```python
from build123d import *

# Parameters (mm, degrees)
SKETCH2_R           = 2.1
BOSS_EXTRUDE1_DEPTH = 4
BOSS_EXTRUDE2_DEPTH = 2
CHAMFER1_SIZE       = 30
CHAMFER1_SIZE2      = 3.683536827087146
FILLET2_R           = 1.5
FILLET4_R           = 1.5


with BuildPart() as part:
    # Sketch2 → Boss-Extrude1 (new body)
    with BuildSketch(Plane(origin=(0, 0, 0), x_dir=(1, 0, 0), z_dir=(0, 1, 0))):
        with BuildLine():
            Line((-4.4, -1.507e-14), (-4.4, 12))
            ThreePointArc((-4.4, 12), (2.7e-16, 16.4), (4.4, 12))
            Line((4.4, 12), (4.4, 1.507e-14))
            Line((4.4, 1.507e-14), (4.4, -38.000000000000014))
            Line((4.4, -38.000000000000014), (-4.399999999999994, -38.000000000000014))
            Line((-4.399999999999994, -38.000000000000014), (-4.4, -1.507e-14))
        make_face()
        with Locations(Location((0, 5, 0), (0, 0, 270))):
            Circle(SKETCH2_R, mode=Mode.SUBTRACT)
    extrude(amount=BOSS_EXTRUDE1_DEPTH)

    # Sketch3 → Boss-Extrude2 (add)
    with BuildSketch(Plane(origin=(0, 4, 0), x_dir=(1, 0, 0), z_dir=(0, 1, 0))):
        Polygon((-12, 0), (12, 0), (12.000000000000002, -38), (-11.999999999999995, -38), align=None)
    extrude(amount=BOSS_EXTRUDE2_DEPTH)

    # Chamfer1
    chamfer1_edges = [part.edges().sort_by_distance(p)[0] for p in [
        (3.55e-15, 0, 38.000000000000014),
    ]]
    chamfer1_side = [part.faces().sort_by_distance(p)[0] for p in [
        (1.53e-15, 0, 11.756614981879217),
    ]]
    chamfer(chamfer1_edges, length=CHAMFER1_SIZE, length2=CHAMFER1_SIZE2, reference=chamfer1_side[0])

    # Fillet2
    # the kernel refuses this fillet: 1.5 mm, written as the material it adds along each edge
    with BuildSketch(Plane(origin=(-4.399999999999994, 4, 38.000000000000014), x_dir=(-4.14e-15, -1, 0), z_dir=(-1.2e-16, 0, -1))) as fillet2_piece_1_section:
        with BuildLine():
            CenterArc((FILLET2_R, FILLET2_R), FILLET2_R, 180, 89.99999999999977)
            Line((6.22e-15, FILLET2_R), (0, 0))
            Line((0, 0), (FILLET2_R, 0))
        make_face()
    fillet2_piece_1 = extrude(amount=38.000000000000014, mode=Mode.PRIVATE)
    fillet2_piece_1 = split(fillet2_piece_1, bisect_by=Plane(origin=(-4.741166225178414, 1.3298279167086908, 18.830579243267316), z_dir=(0, 0.992546151641322, -0.12186934340514775)), keep=Keep.TOP, mode=Mode.PRIVATE)
    add(fillet2_piece_1)
    with BuildSketch(Plane(origin=(4.4, 4, 0), x_dir=(0, -1, 0), z_dir=(0, 0, 1))) as fillet2_piece_2_section:
        with BuildLine():
            CenterArc((FILLET2_R, FILLET2_R), FILLET2_R, 180, 90)
            Line((0, FILLET2_R), (0, 0))
            Line((0, 0), (FILLET2_R, 0))
        make_face()
    fillet2_piece_2 = extrude(amount=38.000000000000014, mode=Mode.PRIVATE)
    fillet2_piece_2 = split(fillet2_piece_2, bisect_by=Plane(origin=(4.741166225178429, 1.3298279167086202, 18.830579243266737), z_dir=(0, 0.992546151641322, -0.12186934340514775)), keep=Keep.TOP, mode=Mode.PRIVATE)
    add(fillet2_piece_2)
    # the kernel refuses this fillet: 1.5 mm, written as the material it takes off along each edge
    with BuildSketch(Plane(origin=(-11.999999999999995, 4, 41.75), x_dir=(0, 1, 0), z_dir=(-1.4e-16, 0, -1))) as fillet2_2_piece_1:
        with BuildLine():
            CenterArc((FILLET2_R, FILLET2_R), FILLET2_R, 180, 90)
            Line((0, FILLET2_R), (0, 0))
            Line((0, 0), (FILLET2_R, 0))
        make_face()
    extrude(amount=45.5, mode=Mode.SUBTRACT)
    with BuildSketch(Plane(origin=(12, 4, -3.75), x_dir=(-1, 0, 5e-17), z_dir=(5e-17, 0, 1))) as fillet2_2_piece_2:
        with BuildLine():
            CenterArc((FILLET2_R, -FILLET2_R), FILLET2_R, 90, 90)
            Line((0, -FILLET2_R), (0, 0))
            Line((0, 0), (FILLET2_R, 0))
        make_face()
    extrude(amount=45.5, mode=Mode.SUBTRACT)

    # Fillet4
    fillet4_edges = [part.edges().sort_by_distance(p)[0] for p in [
        (5.41281689306181, 3.918679886483928, 38),
        (8.2, 4, 38),
        (11.560660171779821, 4.439339828220179, 38),
        (-5.41281689306181, 3.918679886483928, 38),
        (-8.200000000000001, 4, 38),
        (-11.560660171779821, 4.439339828220179, 38),
        (12.000000000000002, 5.75, 38),
        (-11.999999999999995, 5.75, 38),
    ]]
    fillet(fillet4_edges, radius=FILLET4_R)


solid = part.part
```
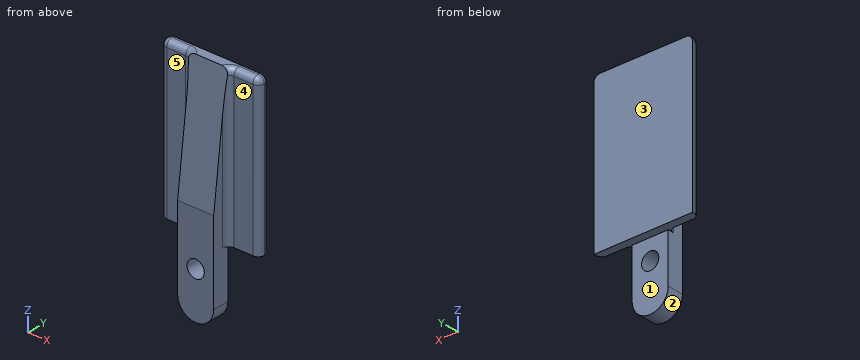
Work out the finished part from the listing and answer in its coordinate system (mm). Face numbers are marked on the shaded views. A direction names the side the tool comes from. Round coordinates to 2 decimals unless told otherwise and drop trailing zeros. Loops run counter-clockwise (first coordinate to the right, second up) from the corner with the lowest first, then second, coordinate; pieces in that order, holes last. Notation, with made-up numbers: (55, -9) -> (76, -9) arc R14 ccw to (76, 11) -> close; hole circle Ø6 at (4, 75). An arc over 180 degrees is marked (long way). Write each question's results on one line, items separated by ' | '. Start each with the question number.
1. Section A-A (x = 0) is taken. Determine the outline of the cut face in (y, z), plus the area to 3 significant figures.
2. A tool of negligible diameter and unlimited length cuts with its end or side. For the marked faces 1, 2, 3, 4 and 5, from which of +Z, -Z, +X, -X, +Y, -Y can it reach the whole face along a straight path? Write none if from no direction.
3. Find the intervals of material crossed by probe 1 along X at (y, z) = (2.35, -5); probe 2 along Y at (x, z) = (-7.5, 18.5); probe 3 along X at (y, z) = (3.5, 2), in increasing order. Write a range as from..to.
4. Section D-D (y = 0.5) is taken. Determine the outline of the cut face in (x, z).
5. Section B-B (z = -5) is taken. Determine the outline of the cut face in (x, y).
6. Section C-C (z = 10) is taken. Determine the outline of the cut face in (x, y).
7. Given pin 1 Ø2.5 at (x, z) = (8.5, 14.5) entering from -Y; pin 2 Ø3 at (x, y) = (6, 1) entering from -Z; pin 3 Ø1 at (x, y) = (-6, 4.5) entering from -Z; pin 4 Ø10 at (x, z) = (6.5, 16) entering from -Y, each flat-ended and moving along its own axis, determine where each tip first touches the part or whether it passes through.
Evaluation:
1) outline: (0, -16.4) -> (4, -16.4) -> (4, -7.1) -> (0, -7.1) -> close; (0, -2.9) -> (4, -2.9) -> (4, 0) -> (6, 0) -> (6, 38) -> (3.68, 38) -> (0, 8) -> close | area: 222 mm2
2) face 1: -Z, +X, -X, +Y | face 2: -Z, +Y, -Y | face 3: +Z, -Z, +X, -X, +Y | face 4: +Z, -Z, +X, -Y | face 5: +Z, -Z, -X, -Y
3) probe 1: x = -4.4..-2.1, 2.1..4.4 | probe 2: y = 4..6 | probe 3: x = -4.78..4.78
4) outline: (-4.4, -12) arc R4.4 ccw to (4.4, -12) -> (4.4, 12.07) -> (-4.4, 12.07) -> close; hole circle Ø4.2 at (0, -5)
5) outline: (-4.4, 0) -> (-2.1, 0) -> (-2.1, 4) -> (-4.4, 4) -> close; (2.1, 0) -> (4.4, 0) -> (4.4, 4) -> (2.1, 4) -> close
6) outline: (-12, 5.5) arc R1.5 ccw to (-10.5, 4) -> (-5.9, 4) arc R1.5 cw to (-4.4, 2.5) -> (-4.4, 0.25) -> (4.4, 0.25) -> (4.4, 2.5) arc R1.5 cw to (5.9, 4) -> (10.5, 4) arc R1.5 ccw to (12, 5.5) -> (12, 6) -> (-12, 6) -> close
7) pin 1: stops at y = 4 | pin 2: passes through | pin 3: stops at z = 0 | pin 4: stops at y = 0.43
